Check sheet for the drawn part. Datum: minimum x, y, z corner. Units: mm. A direction names the side the tool comes from. Round coordinates to 2 decimals unless told otherwise and drop trailing zeros. Order: outer loops, then holes, each group sorted by start corner. A loop starts at its lowest first (then second) coordinate and runs counter-clockwise, first axis right, second up.
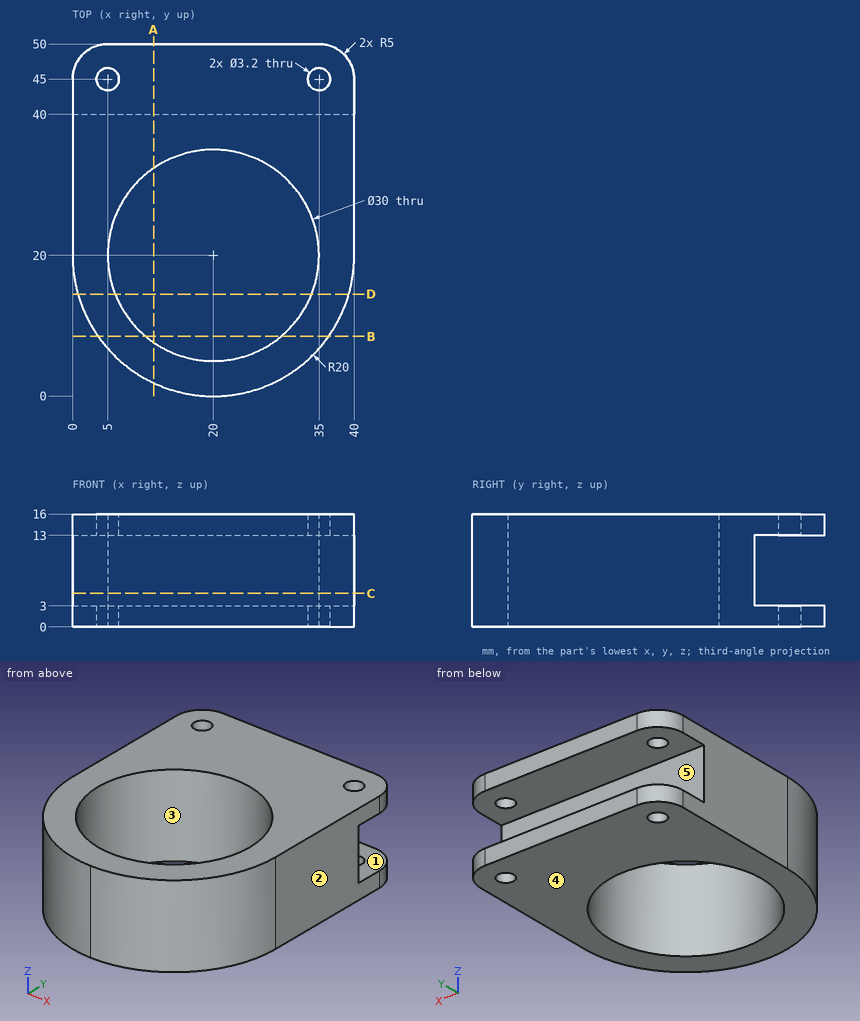
(1) Draft check along X on the marked faces 1, 2 and 3. Enter one of: released by +X, released by -X, zero draft, split by the parting line, or undercut.
Returned:
face 1: zero draft
face 2: released by +X
face 3: undercut
(2) Depth check by flat-ended pin: P1, Ø6, axis at x = 13.5, y = 10.5, coming from the -Z side; P2, Ø5, axis at x = 16, z = 9, coming from the +Y side. Enter the tip coordinate at first touch or a pass-through.
Returned:
P1: passes through
P2: stops at y = 40
(3) Sectioned sample at A-A, the plane x = 11.5. Record the cut outline in (y, z).
Returned:
outline: (1.9, 0) - (7.64, 0) - (7.64, 16) - (1.9, 16) - close; (32.36, 0) - (50, 0) - (50, 3) - (40, 3) - (40, 13) - (50, 13) - (50, 16) - (32.36, 16) - close
(4) Sectioned sample at C-C, the plane z = 4.75. Record the cut outline in (x, y).
Returned:
outline: (0, 20) arc R20 ccw to (40, 20) - (40, 40) - (0, 40) - close; hole circle Ø30 at (20, 20)
(5) Material ranges on line 1 (X direction, y = 45, z = 14.1); line 2 (Y direction, x = 20, z = 5.5); line 3 (Z direction, x = 10, y = 47.5), recorded low to high.
Returned:
line 1: x = 0 to 3.4, 6.6 to 33.4, 36.6 to 40
line 2: y = 0 to 5, 35 to 40
line 3: z = 0 to 3, 13 to 16
(6) Sectioned sample at B-B, the plane y = 8.5. Record the cut outline in (x, z), and give its area (3 significant figures).
Returned:
outline: (3.64, 0) - (10.37, 0) - (10.37, 16) - (3.64, 16) - close; (29.63, 0) - (36.36, 0) - (36.36, 16) - (29.63, 16) - close
area: 215 mm2
(7) Sectioned sample at D-D, the plane y = 14.5. Record the cut outline in (x, z), and give its area (3 significant figures).
Returned:
outline: (0.77, 0) - (6.04, 0) - (6.04, 16) - (0.77, 16) - close; (33.96, 0) - (39.23, 0) - (39.23, 16) - (33.96, 16) - close
area: 169 mm2
(8) Set-up check for the marked faces 4 and 5: record each of +Z, -Z, +X, -X, +Y, -Y from which the full face is reachable in a straight line by a thin tool's end or side.
Returned:
face 4: -Z, +X, -X, +Y, -Y
face 5: +X, -X, +Y
